For this review, take the finished solid that the model builds, in its own axes (mm). A direction names the side the tool comes from. Coordinates: 2 decimals unless noted, no trailing zeros. Loops run counter-clockwise (first coordinate to the right, second up) from the corner with the lowest first, then second, coordinate; pieces in that order, holes last.
1. To check wall thickness, follow probe 1 along X at (y, z) = (52.5, 3.5); probe 2 along X at (y, z) = (63.5, 6.25); probe 3 along X at (y, z) = (62.5, 2). State the ranges of each line that lie inside material, in increasing order.
2. Take a section at C-C, the plane y = 62.5. State the section outline as (x, z) points.
3. Machinability: for faces 1 (the face through (9.958, 51, 4)), 2 (the face through (-12, 56, 0)), 3 (the face through (12, 48.944, 4)), which of the approach directions +Z, -Z, +X, -X, +Y, -Y give a long, thin tool a straight path to every point of the face, cutting with its end or side? Answer none if there is none.
4. Clearance check with flat-ended pins moving along their axes: P1, Ø4, axis at x = -28.5, y = 56, coming from the -Z side; P2, Ø3.5, axis at x = 12, z = 4, coming from the -Y side; P3, Ø2, axis at x = 10, z = 2.5, coming from the +Y side; P4, Ø4, axis at y = 63, z = 3.5, coming from the -X side. State where each tip first meets the part, or that it passes through.
5. Mouldability with a two-part tool opening along X and no side actions: class faces 4 (the face through (8, 53.346, 4)), 5 (the face through (15.402, 49.725, 3.757)), 6 (the face through (-11, 45.478, 4)) as pulls with the +X half, pulls with the -X half, needs draft (parallel to the pull), parting line crosses it, or undercut.
6. Take a section at A-A, the plane z = 2.25. State the section outline as (x, y) points (3 decimals).
7. Take a section at B-B, the plane x = 11.5. State the section outline as (y, z) points, then the cut area to 3 significant figures.
Autodesk Inventor part; units mm, degrees
ref_plane "YZ Plane" through (0, 0, 0) normal (1, 0, 0) x (0, 1, 0)
ref_plane "XZ Plane" through (0, 0, 0) normal (0, 1, 0) x (-1, 0, 0)
ref_plane "XY Plane" through (0, 0, 0) normal (0, 0, 1) x (1, 0, 0)
sketch "Sketch1" plane through (0, 0, 0) normal (0, 0, 1) x (1, 0, 0)
  line L0 (-91.2456, 87.8277) -> (124.6544, 87.8277) construction
  line L1 (124.6544, 87.8277) -> (124.6544, -191.7916) construction
  line L2 (124.6544, -191.7916) -> (-91.2456, -191.7916) construction
  line L3 (-91.2456, -191.7916) -> (-91.2456, 87.8277) construction
  line L4 (-40.6804, 60.9272) -> (-30.3811, 66.9352)
  line L5 (-30.3811, 66.9352) -> (8.2414, 66.9352)
  line L6 (8.2414, 66.9352) -> (16.7044, 63.9312)
  line L7 (16.7044, 63.9312) -> (16.7044, 50.4848)
  line L8 (16.7044, 50.4848) -> (14.0633, 48.9442)
  line L9 (14.0633, 48.9442) -> (9.958, 48.9442)
  line L10 (9.958, 48.9442) -> (9.958, 53.3458)
  line L11 (9.958, 53.3458) -> (6.954, 53.3458)
  line L12 (6.954, 53.3458) -> (6.954, 45.4782)
  line L13 (6.954, 45.4782) -> (-30.3811, 45.4782)
  line L14 (-40.6804, 51.145) -> (-40.6804, 60.9272)
  line L15 (-30.3811, 45.4782) -> (-40.6804, 51.145)
  point P0 (0, 0)
  dimension "d4" = 215.9
extrude "Extrusion1" add sketch "Sketch1" along normal blind 7.62
properties part number "flatcamera"
Results list:
1. probe 1: x = -40.68 to 6.95, 9.96 to 16.7
1. probe 2: x = -36.27 to 16.7
1. probe 3: x = -37.98 to 16.7
2. outline: (-37.98, 0) - (16.7, 0) - (16.7, 7.62) - (-37.98, 7.62) - close
3. face 1: +Z, -Z, -Y
3. face 2: -Z, +X, -X, +Y, -Y
3. face 3: +Z, -Z, +X, -Y
4. P1: stops at z = 0
4. P2: stops at y = 48.94
4. P3: stops at y = 66.67
4. P4: stops at x = -40.56
5. face 4: undercut
5. face 5: pulls with the +X half
5. face 6: needs draft
6. outline: (-40.68, 51.145) - (-30.381, 45.478) - (6.954, 45.478) - (6.954, 53.346) - (9.958, 53.346) - (9.958, 48.944) - (14.063, 48.944) - (16.704, 50.485) - (16.704, 63.931) - (8.241, 66.935) - (-30.381, 66.935) - (-40.68, 60.927) - close
7. outline: (48.94, 0) - (65.78, 0) - (65.78, 7.62) - (48.94, 7.62) - close
7. area: 128 mm2
